Can you work these out from the model? Positions are in its coordinate system, mm. Face numbers are marked on the shaded views. A direction names the side the tool comes from. Give positions to 0.01 mm unless a question says otherwise; leave off trailing zeros. Loops run counter-clockwise (first coordinate to the right, second up) from the corner with the lowest first, then second, coordinate; pieces in that order, holes last. Notation, with made-up numbers: (26, 29.5) -> (69, 29.5) arc R17 cw to (69, 45.5) -> close; hole circle Ø11 at (12, -8.75). An arc over 180 degrees is marked (long way). One line per question, with ' | ' between items.
from build123d import *

# Parameters (mm, degrees)
SKETCH8_R                     = 12
SKETCH8_R_2                   = 10
BOSS_EXTRUDE5_DEPTH           = 7
BOSS_EXTRUDE5_DRAFT           = 1
BOSS_EXTRUDE7_DEPTH           = 2
BOSS_EXTRUDE7_DRAFT           = 1
BOSS_EXTRUDE7_PROFILE_2_DEPTH = 2
BOSS_EXTRUDE7_PROFILE_2_DRAFT = 1
BOSS_EXTRUDE7_PROFILE_3_DEPTH = 2
BOSS_EXTRUDE7_PROFILE_3_DRAFT = 1
BOSS_EXTRUDE7_PROFILE_4_DEPTH = 2
BOSS_EXTRUDE7_PROFILE_4_DRAFT = 1
BOSS_EXTRUDE7_PROFILE_5_DEPTH = 2
BOSS_EXTRUDE7_PROFILE_5_DRAFT = 1
BOSS_EXTRUDE7_PROFILE_6_DEPTH = 2
BOSS_EXTRUDE7_PROFILE_6_DRAFT = 1
BOSS_EXTRUDE7_PROFILE_7_DEPTH = 2
BOSS_EXTRUDE7_PROFILE_7_DRAFT = 1
FILLET3_R                     = 0.2
FILLET4_R                     = 1


with BuildPart() as part:
    # Sketch8 → Boss-Extrude5 (with draft: the straight prism first)
    with BuildSketch(Plane(origin=(0, 0, 0), x_dir=(1, 0, 0), z_dir=(0, 1, 0))):
        with Locations((-0.689500998, 0.229833666)):
            Circle(SKETCH8_R)
        with Locations((-0.689500998, 0.229833666)):
            Circle(SKETCH8_R_2, mode=Mode.SUBTRACT)
    extrude(amount=BOSS_EXTRUDE5_DEPTH)
    # Boss-Extrude5: the draft: its side faces are tilted about the plane it starts from
    boss_extrude5_sides = [part.faces().sort_by_distance(p)[0] for p in [
        (-12.689500998, 3.5, -0.229833666),
        (-10.689500998, 3.5, -0.229833666),
    ]]
    draft(boss_extrude5_sides, Plane(origin=(0, 0, 0), x_dir=(1, 0, 0), z_dir=(0, 1, 0)), BOSS_EXTRUDE5_DRAFT)


with BuildPart() as boss_extrude7_tool:
    # Sketch9 → Boss-Extrude7 (with draft: the straight prism first)
    with BuildSketch(Plane(origin=(0, 7, 0), x_dir=(1, 0, 0), z_dir=(0, 1, 0))):
        with BuildLine():
            ThreePointArc((-7.209347937, -7.512919996), (-7.765123044, -7.008550894), (-8.28199938, -6.464388222))
            Line((-8.28199938, -6.464388222), (-9.545268932, -7.685837669))
            ThreePointArc((-9.545268932, -7.685837669), (-8.992344967, -8.264002947), (-8.401756366, -8.803637179))
            Line((-8.401756366, -8.803637179), (-7.209347937, -7.512919996))
        make_face()
    extrude(amount=BOSS_EXTRUDE7_DEPTH)
    # Boss-Extrude7: the draft: its side faces are tilted about the plane it starts from
    boss_extrude7_sides = [boss_extrude7_tool.faces().sort_by_distance(p)[0] for p in [
        (-8.992344967, 8, 8.264002947),
        (-7.805552152, 8, 8.158278588),
        (-7.765123044, 8, 7.008550894),
        (-8.913634156, 8, 7.075112945),
    ]]
    draft(boss_extrude7_sides, Plane(origin=(0, 7, 0), x_dir=(1, 0, 0), z_dir=(0, 1, 0)), BOSS_EXTRUDE7_DRAFT)


with BuildPart() as part_1:
    add(part.part)

    # Boss-Extrude7: add boss_extrude7_tool
    add(boss_extrude7_tool.part)


with BuildPart() as boss_extrude7_profile_2_tool:
    # Sketch9 → Boss-Extrude7 profile 2 (with draft: the straight prism first)
    with BuildSketch(Plane(origin=(0, 7, 0), x_dir=(1, 0, 0), z_dir=(0, 1, 0))):
        with BuildLine():
            ThreePointArc((-10.809530951, 0.438716694), (-10.761410839, 1.237440003), (-10.650350336, 2.029866676))
            Line((-10.650350336, 2.029866676), (-12.401922464, 2.205096122))
            ThreePointArc((-12.401922464, 2.205096122), (-12.508319943, 1.412202953), (-12.56110308, 0.61394614))
            Line((-12.56110308, 0.61394614), (-10.809530951, 0.438716694))
        make_face()
    extrude(amount=BOSS_EXTRUDE7_PROFILE_2_DEPTH)
    # Boss-Extrude7 profile 2: the draft: its side faces are tilted about the plane it starts from
    boss_extrude7_profile_2_sides = [boss_extrude7_profile_2_tool.faces().sort_by_distance(p)[0] for p in [
        (-11.685317015, 8, -0.526331417),
        (-10.761410839, 8, -1.237440003),
        (-11.5261364, 8, -2.117481399),
        (-12.508319943, 8, -1.412202953),
    ]]
    draft(boss_extrude7_profile_2_sides, Plane(origin=(0, 7, 0), x_dir=(1, 0, 0), z_dir=(0, 1, 0)), BOSS_EXTRUDE7_PROFILE_2_DRAFT)


with BuildPart() as part_2:
    add(part_1.part)

    # Boss-Extrude7 profile 2: add boss_extrude7_profile_2_tool
    add(boss_extrude7_profile_2_tool.part)


with BuildPart() as boss_extrude7_profile_3_tool:
    # Sketch9 → Boss-Extrude7 profile 3 (with draft: the straight prism first)
    with BuildSketch(Plane(origin=(0, 7, 0), x_dir=(1, 0, 0), z_dir=(0, 1, 0))):
        with BuildLine():
            ThreePointArc((-6.727066623, 8.354268397), (-6.166482087, 8.742254974), (-5.581052028, 9.091626199))
            Line((-5.581052028, 9.091626199), (-6.436662035, 10.624669806))
            ThreePointArc((-6.436662035, 10.624669806), (-7.123347108, 10.214226618), (-7.78084598, 9.758490692))
            Line((-7.78084598, 9.758490692), (-6.727066623, 8.354268397))
        make_face()
    extrude(amount=BOSS_EXTRUDE7_PROFILE_3_DEPTH)
    # Boss-Extrude7 profile 3: the draft: its side faces are tilted about the plane it starts from
    boss_extrude7_profile_3_sides = [boss_extrude7_profile_3_tool.faces().sort_by_distance(p)[0] for p in [
        (-7.253956301, 8, -9.056379545),
        (-6.166482087, 8, -8.742254974),
        (-6.008857032, 8, -9.858148003),
        (-7.123347108, 8, -10.214226618),
    ]]
    draft(boss_extrude7_profile_3_sides, Plane(origin=(0, 7, 0), x_dir=(1, 0, 0), z_dir=(0, 1, 0)), BOSS_EXTRUDE7_PROFILE_3_DRAFT)


with BuildPart() as part_3:
    add(part_2.part)

    # Boss-Extrude7 profile 3: add boss_extrude7_profile_3_tool
    add(boss_extrude7_profile_3_tool.part)


with BuildPart() as boss_extrude7_profile_4_tool:
    # Sketch9 → Boss-Extrude7 profile 4 (with draft: the straight prism first)
    with BuildSketch(Plane(origin=(0, 7, 0), x_dir=(1, 0, 0), z_dir=(0, 1, 0))):
        with BuildLine():
            Line((2.366640727, 11.7077462), (1.926100917, 10.008241767))
            ThreePointArc((1.926100917, 10.008241767), (2.578394525, 9.809995315), (3.215863804, 9.568289863))
            Line((3.215863804, 9.568289863), (3.880694044, 11.193217982))
            ThreePointArc((3.880694044, 11.193217982), (3.132335987, 11.475990362), (2.366640727, 11.7077462))
        make_face()
    extrude(amount=BOSS_EXTRUDE7_PROFILE_4_DEPTH)
    # Boss-Extrude7 profile 4: the draft: its side faces are tilted about the plane it starts from
    boss_extrude7_profile_4_sides = [boss_extrude7_profile_4_tool.faces().sort_by_distance(p)[0] for p in [
        (3.132335987, 8, -11.475990362),
        (2.146370822, 8, -10.857993984),
        (2.578394525, 8, -9.809995315),
        (3.548278924, 8, -10.380753922),
    ]]
    draft(boss_extrude7_profile_4_sides, Plane(origin=(0, 7, 0), x_dir=(1, 0, 0), z_dir=(0, 1, 0)), BOSS_EXTRUDE7_PROFILE_4_DRAFT)


with BuildPart() as part_4:
    add(part_3.part)

    # Boss-Extrude7 profile 4: add boss_extrude7_profile_4_tool
    add(boss_extrude7_profile_4_tool.part)


with BuildPart() as boss_extrude7_profile_5_tool:
    # Sketch9 → Boss-Extrude7 profile 5 (with draft: the straight prism first)
    with BuildSketch(Plane(origin=(0, 7, 0), x_dir=(1, 0, 0), z_dir=(0, 1, 0))):
        with BuildLine():
            Line((10.198955387, 4.975778875), (8.561854638, 4.337272925))
            ThreePointArc((8.561854638, 4.337272925), (8.840763983, 3.640506293), (9.06727997, 2.92498923))
            Line((9.06727997, 2.92498923), (10.737769949, 3.470197392))
            ThreePointArc((10.737769949, 3.470197392), (10.493728209, 4.232065904), (10.198955387, 4.975778875))
        make_face()
    extrude(amount=BOSS_EXTRUDE7_PROFILE_5_DEPTH)
    # Boss-Extrude7 profile 5: the draft: its side faces are tilted about the plane it starts from
    boss_extrude7_profile_5_sides = [boss_extrude7_profile_5_tool.faces().sort_by_distance(p)[0] for p in [
        (10.493728209, 8, -4.232065904),
        (9.380405013, 8, -4.6565259),
        (8.840763983, 8, -3.640506293),
        (9.90252496, 8, -3.197593311),
    ]]
    draft(boss_extrude7_profile_5_sides, Plane(origin=(0, 7, 0), x_dir=(1, 0, 0), z_dir=(0, 1, 0)), BOSS_EXTRUDE7_PROFILE_5_DRAFT)


with BuildPart() as part_5:
    add(part_4.part)

    # Boss-Extrude7 profile 5: add boss_extrude7_profile_5_tool
    add(boss_extrude7_profile_5_tool.part)


with BuildPart() as boss_extrude7_profile_6_tool:
    # Sketch9 → Boss-Extrude7 profile 6 (with draft: the straight prism first)
    with BuildSketch(Plane(origin=(0, 7, 0), x_dir=(1, 0, 0), z_dir=(0, 1, 0))):
        with BuildLine():
            Line((9.809829479, -5.324132297), (8.289916221, -4.44228628))
            ThreePointArc((8.289916221, -4.44228628), (7.919054516, -5.094770576), (7.500866623, -5.717982455))
            Line((7.500866623, -5.717982455), (8.968653964, -6.684103064))
            ThreePointArc((8.968653964, -6.684103064), (9.412154061, -6.018289528), (9.809829479, -5.324132297))
        make_face()
    extrude(amount=BOSS_EXTRUDE7_PROFILE_6_DEPTH)
    # Boss-Extrude7 profile 6: the draft: its side faces are tilted about the plane it starts from
    boss_extrude7_profile_6_sides = [boss_extrude7_profile_6_tool.faces().sort_by_distance(p)[0] for p in [
        (9.04987285, 8, 4.883209289),
        (7.919054516, 8, 5.094770576),
        (8.234760293, 8, 6.20104276),
        (9.412154061, 8, 6.018289528),
    ]]
    draft(boss_extrude7_profile_6_sides, Plane(origin=(0, 7, 0), x_dir=(1, 0, 0), z_dir=(0, 1, 0)), BOSS_EXTRUDE7_PROFILE_6_DRAFT)


with BuildPart() as part_6:
    add(part_5.part)

    # Boss-Extrude7 profile 6: add boss_extrude7_profile_6_tool
    add(boss_extrude7_profile_6_tool.part)


with BuildPart() as boss_extrude7_profile_7_tool:
    # Sketch9 → Boss-Extrude7 profile 7 (with draft: the straight prism first)
    with BuildSketch(Plane(origin=(0, 7, 0), x_dir=(1, 0, 0), z_dir=(0, 1, 0))):
        with BuildLine():
            ThreePointArc((1.280752997, -9.698748185), (0.534166556, -9.818115184), (-0.219247003, -9.881422416))
            Line((-0.219247003, -9.881422416), (-0.050535252, -11.630781881))
            ThreePointArc((-0.050535252, -11.630781881), (0.746403959, -11.560868405), (1.536829397, -11.437468136))
            Line((1.536829397, -11.437468136), (1.280752997, -9.698748185))
        make_face()
    extrude(amount=BOSS_EXTRUDE7_PROFILE_7_DEPTH)
    # Boss-Extrude7 profile 7: the draft: its side faces are tilted about the plane it starts from
    boss_extrude7_profile_7_sides = [boss_extrude7_profile_7_tool.faces().sort_by_distance(p)[0] for p in [
        (1.408791197, 8, 10.568108161),
        (0.534166556, 8, 9.818115184),
        (-0.134891127, 8, 10.756102148),
        (0.746403959, 8, 11.560868405),
    ]]
    draft(boss_extrude7_profile_7_sides, Plane(origin=(0, 7, 0), x_dir=(1, 0, 0), z_dir=(0, 1, 0)), BOSS_EXTRUDE7_PROFILE_7_DRAFT)


with BuildPart() as part_7:
    add(part_6.part)

    # Boss-Extrude7 profile 7: add boss_extrude7_profile_7_tool
    add(boss_extrude7_profile_7_tool.part)

    # Fillet3
    fillet3_edges = [part_7.edges().sort_by_distance(p)[0] for p in [
        (-8.967942047, 9, 8.239038679),
        (0.742183685, 9, 11.526214308),
        (9.382464248, 9, 5.999925646),
        (10.460859537, 9, -4.220302928),
        (3.121321399, 9, -11.44286259),
        (-7.104320002, 9, -10.184957078),
        (-12.473583207, 9, -1.408727847),
    ]]
    fillet(fillet3_edges, radius=FILLET3_R)

    # Fillet4
    fillet4_edges = [part_7.edges().sort_by_distance(p)[0] for p in [
        (-6.18550884, 9, -8.771524863),
        (-10.796147575, 9, -1.240915109),
        (-7.789525964, 9, 7.033515162),
        (0.538386829, 9, 9.852769281),
        (7.948744329, 9, 5.113134459),
        (8.873632654, 9, -3.652269269),
        (2.589409961, 9, -9.843123094),
    ]]
    fillet(fillet4_edges, radius=FILLET4_R)


solid = part_7.part
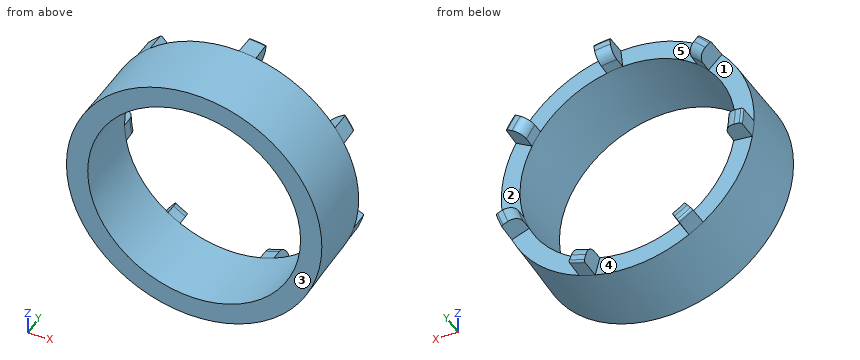
Q1. On a 3-axis mill with a long thin cutter (end or side, diameter ignored), from which of +Z, -Z, +X, -X, +Y, -Y can I reach the whole of each face in a straight line? I mean the marked faces 3, 4 and 5. Say none if no direction works.
Entries:
face 3: +Z, -Z, +X, -X, -Y | face 4: -Z, +Y | face 5: +Z, +Y
Q2. If we section it at C-C (y = 4): Write out the boundary of the cut face in (x, z).
Entries:
outline: circle Ø23.86 at (-0.69, -0.23); hole circle Ø20.14 at (-0.69, -0.23)
Q3. For pin 1 Ø1.2 at (x, z) = (-5.5, 10) entering from +Y; pin 2 Ø4 at (y, z) = (3, 2) entering from +X; pin 3 Ø5 at (x, y) = (-2, 4.5) entering from +Z, each with a flat end and sliding along its axis, tell me the tip position at first contact or that it passes through.
Entries:
pin 1: y = 7 | pin 2: x = 11.27 | pin 3: z = 11.73
Q4. If we section it at A-A (y = 7.5): Write out the boundary of the cut face in (x, z).
Entries:
outline: (-12.55, -0.62) arc R11.87 ccw to (-12.39, -2.2) -> (-10.66, -2.02) arc R10.13 cw to (-10.82, -0.45) -> close; (-9.53, 7.69) -> (-8.28, 6.48) arc R10.13 cw to (-7.22, 7.51) -> (-8.4, 8.79) arc R11.87 ccw to start; (-7.77, -9.76) arc R11.87 ccw to (-6.44, -10.61) -> (-5.59, -9.1) arc R10.13 cw to (-6.73, -8.37) -> close; (-0.21, 9.89) arc R10.13 cw to (1.27, 9.71) -> (1.53, 11.43) arc R11.87 ccw to (-0.04, 11.62) -> close; (1.94, -10.01) -> (2.37, -11.7) arc R11.87 ccw to (3.87, -11.19) -> (3.21, -9.58) arc R10.13 cw to start; (7.51, 5.72) arc R10.13 cw to (8.29, 4.45) -> (9.8, 5.33) arc R11.87 ccw to (8.97, 6.67) -> close; (8.57, -4.33) -> (10.19, -4.96) arc R11.87 ccw to (10.73, -3.48) -> (9.07, -2.94) arc R10.13 cw to start
Q5. If we section it at B-B (y = 6): Write out the boundary of the cut face in (x, z), plus the area to 3 significant figures.
Entries:
outline: circle Ø23.79 at (-0.69, -0.23); hole circle Ø20.21 at (-0.69, -0.23) | area: 124 mm²
Q6. If I drill on probe 1 along X at (y, z) = (2.5, -2.5); probe 2 along X at (y, z) = (6.5, -8.5); probe 3 along Z at (x, y) = (1.75, 6.5) (3 decimals), over which ranges is the centre line in solid material (lowest first)? Write a range as from..to.
Entries:
probe 1: -12.43..-10.47, 9.09..11.05 | probe 2: -9.23..-6.51, 5.13..7.85 | probe 3: -11.863..-10.045, 9.585..11.404
Q7. If we mould it in two halves opening along Z, with no side actions, what happens to the marked faces 1 and 2? For each: pulls with the +Z half, pulls with the -Z half, needs draft (parallel to the pull), parting line crosses it, or undercut.
Entries:
face 1: needs draft | face 2: undercut
